from build123d import *

# Parameters (mm, degrees)
CYLINDER035_R     = 5
CYLINDER035_DEPTH = 15
CYLINDER034_R     = 5
CYLINDER034_DEPTH = 16
BOX017_W          = 19
BOX017_H          = 18
BOX017_DEPTH      = 19.5
FILLET006_R       = 8.5


with BuildPart() as c_top_hole001:
    # Cylinder035 → Cylinder035 (new body)
    with BuildSketch(Plane(origin=(-5, 0, 11.5), x_dir=(0, 0, -1), z_dir=(1, 0, 0))):
        Circle(CYLINDER035_R)
    extrude(amount=CYLINDER035_DEPTH)


with BuildPart() as c_holes:
    # Cylinder034 → Cylinder034 (new body)
    with BuildSketch(Plane.XY):
        Circle(CYLINDER034_R)
    extrude(amount=CYLINDER034_DEPTH)

    # Fusion039: union C-Top-Hole001
    add(c_top_hole001.part)


with BuildPart() as corner:
    # Box017 → Box017 (new body)
    with BuildSketch(Plane(origin=(-9, -9.5, 0), x_dir=(1, 0, 0), z_dir=(0, 0, 1))):
        with Locations((9.5, 9)):
            Rectangle(BOX017_W, BOX017_H)
    extrude(amount=BOX017_DEPTH)

    # Fillet006
    fillet006_edges = [corner.edges().sort_by_distance(p)[0] for p in [
        (-9, -9.5, 9.75),
        (-9, -0.5, 19.5),
        (-9, 8.5, 9.75),
        (0.5, -9.5, 19.5),
        (0.5, 8.5, 19.5),
    ]]
    fillet(fillet006_edges, radius=FILLET006_R)

    # Cut: cut C-Holes
    add(c_holes.part, mode=Mode.SUBTRACT)


solid = corner.part
Model file for the job. Use its own axes, mm. A direction names the side the tool comes from. Give positions to 0.01 mm unless a question says otherwise; leave off trailing zeros. Order: outer loops, then holes, each group sorted by start corner. A loop starts at its lowest first (then second) coordinate and runs counter-clockwise, first axis right, second up. Notation, with made-up numbers: (41.5, -30) - (96.5, -30) arc R24 ccw to (96.5, -8) - close; hole circle Ø9 at (-7, 61). An arc over 180 degrees is marked (long way). Return JSON: item names as keys, results as strings.
1) Flat gauge pins, fed straight in: P1, Ø6, axis at x = -4.5, y = 0.5, coming from the +Z side; P2, Ø2.5, axis at x = -2, y = -3, coming from the -Z side; P3, Ø6, axis at y = -5, z = 7, coming from the -X side. Where does each tip first touch, or does it go through?
Geometry says:
{"P1": "z = 19.44", "P2": "z = 16", "P3": "x = -8.94"}
2) Cut at C-C, the plane z = 14.25. Give the cut face in (x, y), plus the area to 3 significant figures.
Geometry says:
{"outline": "(-8.35, -1) arc R7.85 ccw to (-0.5, -8.85) - (10, -8.85) - (10, -4.18) - (2.75, -4.18) arc R5 cw to (-2.75, -4.18) - (-5, -4.18) - (-5, 4.18) - (-2.75, 4.18) arc R5 cw to (2.75, 4.18) - (10, 4.18) - (10, 7.85) - (-0.5, 7.85) arc R7.85 ccw to (-8.35, 0) - close", "area": "149 mm²"}
3) Cut at B-B, the plane x = 6.5. Give the cut face in (y, z), plus the area to 3 significant figures.
Geometry says:
{"outline": "(-9.5, 0) - (8.5, 0) - (8.5, 11) arc R8.5 ccw to (0, 19.5) - (-1, 19.5) arc R8.5 ccw to (-9.5, 11) - close; hole circle Ø10 at (0, 11.5)", "area": "241 mm²"}
4) Cut at D-D, the plane y = -7.75. Give the cut face in (x, z).
Geometry says:
{"outline": "(-5.67, 0) - (10, 0) - (10, 16.17) - (-0.5, 16.17) arc R5.17 ccw to (-5.67, 11) - close"}
5) 3-axis set-ups, long thin cutter, end or side, ignore diameter. For faces 1 (the cylindrical face through (0, -5, 15)), 2 (the flat face through (-5, 0, 12)), 3 (the flat face through (-9, -0.5, 5.4)): which of +Z, -Z, +X, -X, +Y, -Y reach the whole face in a straight line?
Geometry says:
{"face 1": "-Z", "face 2": "+X", "face 3": "+Z, -Z, -X, +Y, -Y"}
6) Cut at A-A, the plane z = 6. Give the cut face in (x, y).
Geometry says:
{"outline": "(-9, -1) arc R8.5 ccw to (-0.5, -9.5) - (10, -9.5) - (10, 8.5) - (-0.5, 8.5) arc R8.5 ccw to (-9, 0) - close; hole circle Ø10 at (0, 0)"}
7) Probe line 1 (Y direction, x = 0, z = 5.5); line 2 (Y direction, x = 4.75, z = 10.5); line 3 (X direction, y = -1.25, z = 1.25). List the from-to ranges inside material, lowest first. Write a range as from..to.
Geometry says:
{"line 1": "-9.5..-5, 5..8.5", "line 2": "-9.5..-4.9, 4.9..8.5", "line 3": "-9..-4.84, 4.84..10"}
8) Pull direction X, two halves, no side cores. Call faces 4 (the cylindrical face through (0, 5, 15)), 5 (the flat face through (10, -1, 5)), 6 (the flat face through (5, -9.5, 5)): pulls with the +X half, pulls with the -X half, needs draft (parallel to the pull), parting line crosses it, or undercut.
Geometry says:
{"face 4": "undercut", "face 5": "pulls with the +X half", "face 6": "needs draft"}
